For this review, take the finished solid that the model builds, in its own axes (mm). A direction names the side the tool comes from. Coordinates: 2 decimals unless noted, no trailing zeros. Order: outer loops, then holes, each group sorted by start corner. A loop starts at its lowest first (then second) coordinate and runs counter-clockwise, first axis right, second up.
from build123d import *

# Parameters (mm, degrees)
SKETCH_1_W                = 260
SKETCH_1_H                = 120
EXTRUDE_1_DEPTH           = 12
HOLE_WIZARD_M6_1_D        = 5
HOLE_WIZARD_M6_1_DEPTH    = 15
HOLE_WIZARD_M6_1_TIP      = 1.502151548
CUT_EXTRUDE_1_DEPTH       = 144.680200445
HOLE_WIZARD_1_D           = 6.6
HOLE_WIZARD_1_CBORE_D     = 11
HOLE_WIZARD_1_CBORE_DEPTH = 6.8
HOLE_WIZARD_M6_3_D        = 5
HOLE_WIZARD_M6_3_DEPTH    = 15
HOLE_WIZARD_M6_3_TIP      = 1.502151548
HOLE_WIZARD_M5_1_D        = 4.2
HOLE_WIZARD_M6_4_D        = 5
HOLE_WIZARD_M6_5_D        = 5
HOLE_WIZARD_M6_5_DEPTH    = 15
HOLE_WIZARD_M6_5_TIP      = 1.502151548


with BuildPart() as part:
    # 草图1 → 凸台-拉伸1 (new body)
    with BuildSketch(Plane(origin=(0, 0, 0), x_dir=(1, 0, 0), z_dir=(0, 1, 0))):
        Rectangle(SKETCH_1_W, SKETCH_1_H)
    extrude(amount=EXTRUDE_1_DEPTH)

    # M6 螺纹孔1
    with Locations(Plane.XY.offset(60)):
        with Locations((-124, 6), (0, 6), (124, 6)):
            Hole(HOLE_WIZARD_M6_1_D / 2, depth=HOLE_WIZARD_M6_1_DEPTH)
            with Locations((0, 0, -(HOLE_WIZARD_M6_1_DEPTH + HOLE_WIZARD_M6_1_TIP / 2))):  # 118° drill point
                Cone(0, HOLE_WIZARD_M6_1_D / 2, HOLE_WIZARD_M6_1_TIP, mode=Mode.SUBTRACT)

    # 草图4 → 切除-拉伸1 (cut, through all)
    with BuildSketch(Plane(origin=(0, 12, 0), x_dir=(1, 0, 0), z_dir=(0, 1, 0))):
        with BuildLine():
            Line((25.5, -10), (25.5, -20))
            ThreePointArc((25.5, -20), (0, -45.5), (-25.5, -20))
            Line((-25.5, -20), (-25.5, -10))
            ThreePointArc((-25.5, -10), (0, 15.5), (25.5, -10))
        make_face()
    extrude(amount=-CUT_EXTRUDE_1_DEPTH, mode=Mode.SUBTRACT)

    # 打孔尺寸根据内六角圆柱头螺钉的类型1 (through all)
    with Locations(Plane(origin=(0, 12, 0), x_dir=(1, 0, 0), z_dir=(0, 1, 0))):
        with Locations((-35, 38), (35, 38), (0, 38)):
            CounterBoreHole(HOLE_WIZARD_1_D / 2, HOLE_WIZARD_1_CBORE_D / 2, HOLE_WIZARD_1_CBORE_DEPTH)

    # M6 螺纹孔3
    with Locations(Plane(origin=(0, 0, -60), x_dir=(-1, 0, 0), z_dir=(0, 0, -1))):
        with Locations((20, 6), (-20, 6)):
            Hole(HOLE_WIZARD_M6_3_D / 2, depth=HOLE_WIZARD_M6_3_DEPTH)
            with Locations((0, 0, -(HOLE_WIZARD_M6_3_DEPTH + HOLE_WIZARD_M6_3_TIP / 2))):  # 118° drill point
                Cone(0, HOLE_WIZARD_M6_3_D / 2, HOLE_WIZARD_M6_3_TIP, mode=Mode.SUBTRACT)

    # M5 螺纹孔1 (through all)
    with Locations(Plane(origin=(0, 12, 0), x_dir=(1, 0, 0), z_dir=(0, 1, 0))):
        with Locations((37.5, 5), (37.5, -35), (-37.5, -35), (-37.5, 5)):
            Hole(HOLE_WIZARD_M5_1_D / 2)

    # M6 螺纹孔4 (through all)
    with Locations(Plane(origin=(0, 12, 0), x_dir=(1, 0, 0), z_dir=(0, 1, 0))):
        with Locations((50, 6), (-50, 6)):
            Hole(HOLE_WIZARD_M6_4_D / 2)

    # M6 螺纹孔5
    with Locations(Plane(origin=(0, 0, 0), x_dir=(-1, 0, 0), z_dir=(0, -1, 0))):
        with Locations((99, -40), (99, 40), (-99, 40), (-99, -40)):
            Hole(HOLE_WIZARD_M6_5_D / 2, depth=HOLE_WIZARD_M6_5_DEPTH)
            with Locations((0, 0, -(HOLE_WIZARD_M6_5_DEPTH + HOLE_WIZARD_M6_5_TIP / 2))):  # 118° drill point
                Cone(0, HOLE_WIZARD_M6_5_D / 2, HOLE_WIZARD_M6_5_TIP, mode=Mode.SUBTRACT)

    # 草图15 → M4 螺纹孔1 (revolve, cut)
    with BuildSketch(Plane(origin=(-130, 6, -40), x_dir=(0, 0, 1), z_dir=(0, 1, 0))):
        Polygon((0, 0), (0, 11.091420021), (1.65, 10.1), (1.65, 0), align=None)
    hole_wizard_m4_1 = revolve(axis=Axis((-136.35, 6, -40), (1, 0, 0)), mode=Mode.SUBTRACT)

    # 镜向1: M4 螺纹孔1 across plane
    add(hole_wizard_m4_1.mirror(Plane(origin=(0, 0, 0), x_dir=(0, 0, 1), z_dir=(1, 0, 0))), mode=Mode.SUBTRACT)


solid = part.part
1. Take a section at D-D, the plane z = 4. Give the boundary of the cut face in (x, y).
Answer below:
outline: (-130, 0) - (-24.78, 0) - (-24.78, 12) - (-130, 12) - close; (24.78, 0) - (130, 0) - (130, 12) - (24.78, 12) - close
2. Clearance check with a flat-ended pin moving along its axis: pin 1 Ø2 at (y, z) = (6, -40) entering from +X. State where the tip first meets the part, or that it passes through.
Answer below:
pin 1: stops at x = 119.51
3. Machinability: for faces 4 (the face through (121.615, 6.751, 52.395)), 5 (the face through (25.5, 6, 15)), 6 (the face through (-40.495, 8.648, -38.242)), 7 (the face through (130, 6, 1)), which of the approach directions +Z, -Z, +X, -X, +Y, -Y give a long, thin tool a straight path to every point of the face, cutting with its end or side? Answer none if there is none.
Answer below:
face 4: +Z
face 5: +Y, -Y
face 6: +Y
face 7: +Z, -Z, +X, +Y, -Y
4. Take a section at A-A, the plane x = -12. Give the boundary of the cut face in (y, z).
Answer below:
outline: (0, -60) - (12, -60) - (12, -12.5) - (0, -12.5) - close; (0, 42.5) - (12, 42.5) - (12, 60) - (0, 60) - close
5. Take a section at B-B, the plane x = 99. Give the boundary of the cut face in (y, z).
Answer below:
outline: (0, -60) - (12, -60) - (12, -42.5) - (0, -42.5) - close; (0, -37.5) - (12, -37.5) - (12, 37.5) - (0, 37.5) - close; (0, 42.5) - (12, 42.5) - (12, 60) - (0, 60) - close
6. To check wall thickness, follow L1, parallel to X at y = 6, z = 50.25; L2, parallel to X at y = 7, z = 17; L3, parallel to X at y = 2, z = -5.5. State the ranges of each line that lie inside material, in increasing order.
Answer below:
L1: x = -130 to -126.5, -121.5 to -2.5, 2.5 to 121.5, 126.5 to 130
L2: x = -130 to -25.5, 25.5 to 130
L3: x = -130 to -52.45, -47.55 to -39.54, -35.46 to -20.25, 20.25 to 35.46, 39.54 to 47.55, 52.45 to 130
7. The part is to be moulded in two halves that separate along Y. For faces 1 (the face through (0, 5.2, -34)), 2 (the face through (-130, 6, 1)), 3 (the face through (17.5, 6.1, -52.4)), say which applies: +Y half, -Y half, draft (parallel to the pull), parting line (faces both ways), or undercut.
Answer below:
face 1: +Y half
face 2: draft
face 3: undercut
8. Take a section at C-C, the plane z = 40. Give the boundary of the cut face in (x, y).
Answer below:
outline: (-130, 0) - (-101.5, 0) - (-101.5, 12) - (-130, 12) - close; (-96.5, 0) - (-15.82, 0) - (-15.82, 12) - (-96.5, 12) - close; (15.82, 0) - (96.5, 0) - (96.5, 12) - (15.82, 12) - close; (101.5, 0) - (130, 0) - (130, 12) - (101.5, 12) - close
